from build123d import *

# Parameters (mm, degrees)
SKETCH1_W           = 58
SKETCH1_H           = 63
BOSS_EXTRUDE1_DEPTH = 16
SKETCH2_W           = 4.7625
SKETCH2_H           = 6.35
BOSS_EXTRUDE2_DEPTH = 6.35


with BuildPart() as part:
    # Sketch1 → Boss-Extrude1 (new body)
    with BuildSketch(Plane.XY):
        with Locations((29, 31.5)):
            Rectangle(SKETCH1_W, SKETCH1_H)
    extrude(amount=BOSS_EXTRUDE1_DEPTH)

    # Sketch2 → Boss-Extrude2 (add)
    with BuildSketch(Plane.ZY):
        with Locations((2.38125, 47.125)):
            Rectangle(SKETCH2_W, SKETCH2_H)
    extrude(amount=BOSS_EXTRUDE2_DEPTH)


solid = part.part
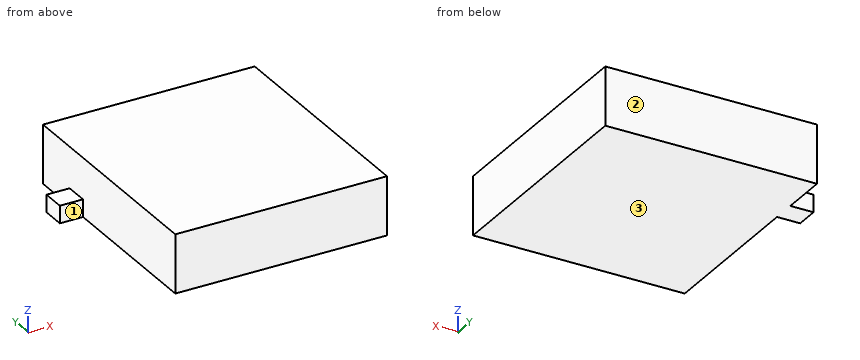
Part model, mm, in its own coordinate system. Face numbers are marked on the shaded views. Coordinates: 2 decimals unless noted, no trailing zeros. Loops run counter-clockwise (first coordinate to the right, second up) from the corner with the lowest first, then second, coordinate; pieces in that order, holes last. Notation, with made-up numbers: M -22,44.5 L 3,44.5 A10 cw 3,56.5 Z; hole C -1.5,32 d3. An arc over 180 degrees is marked long. Use a Markdown table: item, result. Add a question column.
Q1. Cut at B-B (y = 58). Write the cut outline in (x, z).
Q2. Mould opens along Y. For the marked faces 1, 2 and 3 say: +Y half, -Y half, draft (parallel to the pull), parting line (faces both ways), or undercut.
Q3. Probe L1, parallel to X at y = 17.5, z = 5.5; L2, parallel to Y at x = -1.5, z = 2. List the from-to ranges inside material, lowest first.
Q4. Cut at A-A (z = 2.5). Write the cut outline in (x, y).
Q5. Cut at C-C (z = 13.25). Write the cut outline in (x, y), and give its area (3 significant figures).
Q6. Pin check, flat tips, straight feed: P1, Ø1.4, axis at x = -2.5, z = 2.5, coming from the -Y side; P2, Ø4, axis at x = -2.5, z = 2.5, coming from the +Y side; P3, Ø5, axis at y = 37.5, z = 9, coming from the -X side. Stop position of each tip, or through.
Worked out:
| question | item | result |
|---|---|---|
| 1 | outline | M 0,0 L 58,0 L 58,16 L 0,16 Z |
| 2 | face 1 | -Y half |
| 2 | face 2 | +Y half |
| 2 | face 3 | draft |
| 3 | L1 | x = 0 to 58 |
| 3 | L2 | y = 43.95 to 50.3 |
| 4 | outline | M -6.35,43.95 L 0,43.95 L 0,0 L 58,0 L 58,63 L 0,63 L 0,50.3 L -6.35,50.3 Z |
| 5 | outline | M 0,0 L 58,0 L 58,63 L 0,63 Z |
| 5 | area | 3,650 mm2 |
| 6 | P1 | stops at y = 43.95 |
| 6 | P2 | stops at y = 50.3 |
| 6 | P3 | stops at x = 0 |
